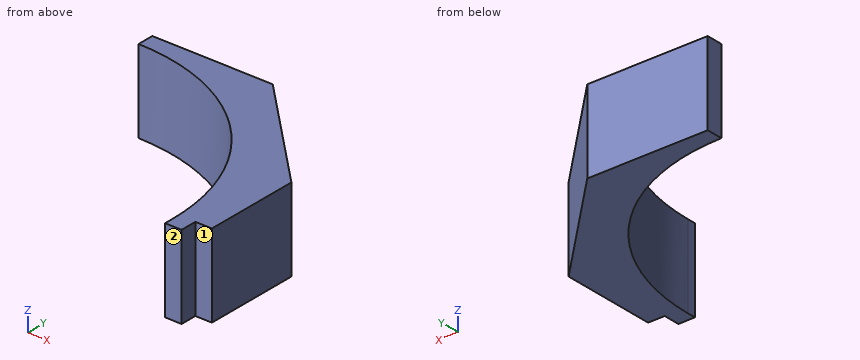
```python
from build123d import *

# Parameters (mm, degrees)
BOSS_EXTRUDE2_DEPTH = 12.7
SKETCH3_W           = 5.08
SKETCH3_H           = 25.4
CUT_EXTRUDE1_DEPTH  = 52.992503306
BOSS_EXTRUDE3_DEPTH = 12.7


with BuildPart() as part:
    # Sketch2 → Boss-Extrude2 (new body)
    with BuildSketch(Plane.XY):
        with BuildLine():
            Line((0, 30.48), (0, 33.02))
            Line((0, 33.02), (18.49751337, 33.02))
            Line((18.49751337, 33.02), (35.56, 15.95751337))
            Line((35.56, 15.95751337), (38.1, -1.27))
            Line((38.1, -1.27), (35.56, -1.27))
            Line((35.56, -1.27), (30.48, -1.27))
            Line((30.48, -1.27), (30.48, 0))
            ThreePointArc((30.48, 0), (21.552614691, 21.552614691), (0, 30.48))
        make_face()
    extrude(amount=BOSS_EXTRUDE2_DEPTH)

    # Sketch3 → Cut-Extrude1 (cut, through all)
    with BuildSketch(Plane.XY.offset(12.7)):
        with Locations((35.56, 11.43)):
            Rectangle(SKETCH3_W, SKETCH3_H)
    extrude(amount=-CUT_EXTRUDE1_DEPTH, mode=Mode.SUBTRACT)

    # Sketch4 → Boss-Extrude3 (add)
    with BuildSketch(Plane.XY.offset(12.7)):
        Polygon((33.02, 1.27), (35.56, 1.27), (35.56, 15.95751337), (33.02, 18.49751337), align=None)
    extrude(amount=-BOSS_EXTRUDE3_DEPTH)


solid = part.part
```
Geometry: final body of the model. Coordinates: model frame, mm. Face numbers are marked on the shaded views. A direction names the side the tool comes from. Round coordinates to 2 decimals unless told otherwise and drop trailing zeros. Order: outer loops, then holes, each group sorted by start corner. A loop starts at its lowest first (then second) coordinate and runs counter-clockwise, first axis right, second up. Notation, with made-up numbers: M 72,17.5 L 103,17.5 A16 ccw 103,24.5 Z; hole C 0.25,-13 d1. An arc over 180 degrees is marked long. One line per item, written item: value.
(1) Reachability of the marked faces 1 and 2 from +Z, -Z, +X, -X, +Y, -Y: full face, straight path, thin tool, end or side. Return the list, or none.
Result sheet:
face 1: +Z, -Z, +X, -Y
face 2: +Z, -Z, +X, -X, -Y
(2) Cut plane A-A (z = 8.25). Return the cut outline in (x, y), and give its area (3 significant figures).
Result sheet:
outline: M 0,30.48 A30.48 cw 30.48,0 L 30.48,-1.27 L 33.02,-1.27 L 33.02,1.27 L 35.56,1.27 L 35.56,15.96 L 18.5,33.02 L 0,33.02 Z
area: 299 mm2
(3) Cut plane B-B (x = 25). Return the cut outline in (y, z), and give its area (3 significant figures).
Result sheet:
outline: M 17.44,0 L 26.52,0 L 26.52,12.7 L 17.44,12.7 Z
area: 115 mm2
(4) Cut plane C-C (y = 17). Return the cut outline in (x, z).
Result sheet:
outline: M 25.3,0 L 34.52,0 L 34.52,12.7 L 25.3,12.7 Z
(5) Line query: probe 1 along X at (y, z) = (26, 8.25); probe 2 along X at (y, z) = (18, 1.25); probe 3 along Y at (x, z) = (34.5, 10.5). Output: solid intervals per line, ascending. Write a range as [from, to].
Result sheet:
probe 1: [15.91, 25.52]
probe 2: [24.6, 33.52]
probe 3: [1.27, 17.02]
(6) Pin query (flat end, axial travel): P1, Ø2, axis at x = 24.5, z = 3, coming from the +Y side; P2, Ø1.3, axis at y = 0.5, z = 3.5, coming from the +X side; P3, Ø3, axis at x = 25.5, z = 5, coming from the -Y side. Return the tip coordinate at first contact, or that it passes through.
Result sheet:
P1: y = 28.02
P2: x = 33.02
P3: y = 14.14
